Part model, mm, in its own coordinate system. Round coordinates to 2 decimals unless told otherwise and drop trailing zeros. Loops run counter-clockwise (first coordinate to the right, second up) from the corner with the lowest first, then second, coordinate; pieces in that order, holes last.
(1) Probe probe 1 along Z at (x, y) = (6, -36.25); probe 2 along X at (y, z) = (-32.75, 1.25); probe 3 along X at (y, z) = (-36.25, 10). List the from-to ranges inside material, lowest first.
(2) Cut at C-C on x = 31. List the corners of the cut face in (y, z), then the cut area to 3 significant figures.
(3) Cut at A-A on z = 9.75. List the corners of the cut face in (x, y).
(4) Cut at B-B on x = -5.5. List the corners of the cut face in (y, z), then the cut area to 3 significant figures.
(5) Flat gauge pins, fed straight in: pin 1 (2 mm diameter, centred on x = -1.5, y = -36.5, fed in from -Z); pin 2 (4 mm diameter, centred on x = 16, y = -29, fed in from +Z); pin 3 (6 mm diameter, centred on x = -14, y = -32, fed in from +Z). Where does each tip first touch, or does it go through?
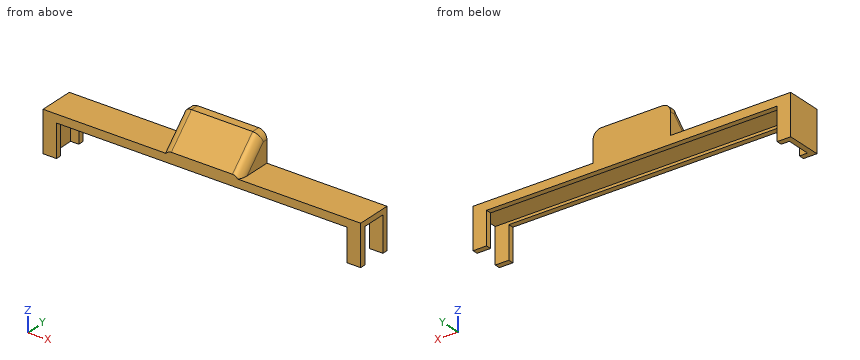
from build123d import *

# Parameters (mm, degrees)
SKETCH1_W           = 117.2
SKETCH1_H           = 13
SKETCH1_W_2         = 113.2
SKETCH1_H_2         = 9
BOSS_EXTRUDE1_DEPTH = 15
SKETCH2_W           = 117.2
SKETCH2_H           = 13
BOSS_EXTRUDE2_DEPTH = 2
SKETCH3_W           = 107.2
SKETCH3_H           = 12
CUT_EXTRUDE1_DEPTH  = 74.389715066
CUT_EXTRUDE2_REACH  = 125.963
SKETCH4_W           = 13
SKETCH4_H           = 9
SKETCH5_W           = 28.56
SKETCH5_H           = 13
BOSS_EXTRUDE3_DEPTH = 11
CHAMFER1_SIZE       = 10
FILLET1_R           = 3
FILLET2_R           = 3


with BuildPart() as part:
    # Sketch1 → Boss-Extrude1 (new body)
    with BuildSketch(Plane.XY):
        with Locations((-12.05444273, -30.99749435)):
            Rectangle(SKETCH1_W, SKETCH1_H)
        with Locations((-12.05444273, -30.99749435)):
            Rectangle(SKETCH1_W_2, SKETCH1_H_2, mode=Mode.SUBTRACT)
    extrude(amount=BOSS_EXTRUDE1_DEPTH)

    # Sketch2 → Boss-Extrude2 (add)
    with BuildSketch(Plane.XY.offset(15)):
        with Locations((-12.05444273, -30.99749435)):
            Rectangle(SKETCH2_W, SKETCH2_H)
    extrude(amount=-BOSS_EXTRUDE2_DEPTH)

    # Sketch3 → Cut-Extrude1 (cut, through all)
    with BuildSketch(Plane.XZ.offset(37.49749435)):
        with Locations((-12.05444273, 6)):
            Rectangle(SKETCH3_W, SKETCH3_H)
    extrude(amount=-CUT_EXTRUDE1_DEPTH, mode=Mode.SUBTRACT)

    # Sketch4 → Cut-Extrude2 (cut, up to next)
    with BuildSketch(Plane(origin=(46.54555727, 0, 0), x_dir=(0, 0, -1), z_dir=(1, 0, 0)), mode=Mode.PRIVATE) as cut_extrude2_sk1:
        with Locations((-6.5, -30.99749435)):
            Rectangle(SKETCH4_W, SKETCH4_H)
    cut_extrude2_tool1 = extrude(cut_extrude2_sk1.sketch, amount=-CUT_EXTRUDE2_REACH, mode=Mode.PRIVATE) & part.part
    add(cut_extrude2_tool1.solids().sort_by_distance((46.545557, -30.997494, 6.5))[0], mode=Mode.SUBTRACT)

    # Sketch5 → Boss-Extrude3 (add)
    with BuildSketch(Plane.XY.offset(15)):
        with Locations((-12.05444273, -30.99749435)):
            Rectangle(SKETCH5_W, SKETCH5_H)
    extrude(amount=BOSS_EXTRUDE3_DEPTH)

    # Chamfer1
    chamfer1_edges = [part.edges().sort_by_distance(p)[0] for p in [
        (-12.05444273, -37.49749435, 26),
    ]]
    chamfer(chamfer1_edges, length=CHAMFER1_SIZE)

    # Fillet1
    fillet1_edges = [part.edges().sort_by_distance(p)[0] for p in [
        (-26.33444273, -25.99749435, 26),
        (-26.33444273, -32.49749435, 21),
    ]]
    fillet(fillet1_edges, radius=FILLET1_R)

    # Fillet2
    fillet2_edges = [part.edges().sort_by_distance(p)[0] for p in [
        (2.22555727, -25.99749435, 26),
        (2.22555727, -32.49749435, 21),
    ]]
    fillet(fillet2_edges, radius=FILLET2_R)


solid = part.part
Final values:
1. probe 1: z = 12 to 15
1. probe 2: x = -70.65 to -68.65
1. probe 3: x = -70.65 to -65.65, 41.55 to 46.55
2. outline: (-37.5, 12) - (-35.5, 12) - (-35.5, 13) - (-26.5, 13) - (-26.5, 12) - (-24.5, 12) - (-24.5, 15) - (-37.5, 15) - close
2. area: 30.0 mm2
3. outline: (-70.65, -37.5) - (-65.65, -37.5) - (-65.65, -35.5) - (-68.65, -35.5) - (-68.65, -26.5) - (-65.65, -26.5) - (-65.65, -24.5) - (-70.65, -24.5) - close; (41.55, -37.5) - (46.55, -37.5) - (46.55, -35.5) - (41.55, -35.5) - close; (41.55, -26.5) - (46.55, -26.5) - (46.55, -24.5) - (41.55, -24.5) - close
4. outline: (-37.5, 12) - (-35.5, 12) - (-35.5, 13) - (-26.5, 13) - (-26.5, 12) - (-24.5, 12) - (-24.5, 26) - (-27.5, 26) - (-37.5, 16) - close
4. area: 123 mm2
5. pin 1: stops at z = 12
5. pin 2: stops at z = 15
5. pin 3: stops at z = 24.5
